```python
from build123d import *

# Parameters (mm, degrees)
SKETCH1_W           = 14.829713536
SKETCH1_H           = 33
SKETCH1_R           = 2
BOSS_EXTRUDE1_DEPTH = 4
BOSS_EXTRUDE2_DEPTH = 24


with BuildPart() as part:
    # Sketch1 → Boss-Extrude1 (new body)
    # profile 1 of 3: a face of its own
    with BuildSketch(Plane.XY):
        with Locations((7.414856768, 16.5)):
            Rectangle(SKETCH1_W, SKETCH1_H)
        with Locations((3, 2.5)):
            Circle(SKETCH1_R, mode=Mode.SUBTRACT)
        with Locations((3, 30.5)):
            Circle(SKETCH1_R, mode=Mode.SUBTRACT)
    # profile 2 of 3: a face of its own
    with BuildSketch(Plane.XY):
        Polygon((14.829713536, 33), (14.829713536, 0), (35.322939572, 0), (35.322939572, 22.058501613), (44.771529769, 22.058501613), (44.771529769, 33), align=None)
    # profile 3 of 3: a face of its own
    with BuildSketch(Plane.XY):
        Polygon((35.322939572, 22.058501613), (35.322939572, 0), (50, 0), (50, 33), (44.771529769, 33), (44.771529769, 22.058501613), align=None)
        with Locations((47, 2.5)):
            Circle(SKETCH1_R, mode=Mode.SUBTRACT)
        with Locations((47, 30.5)):
            Circle(SKETCH1_R, mode=Mode.SUBTRACT)
    extrude(amount=BOSS_EXTRUDE1_DEPTH)

    # Sketch1_3 → Boss-Extrude2 (add)
    with BuildSketch(Plane.XY):
        Polygon((14.829713536, 33), (14.829713536, 0), (35.322939572, 0), (35.322939572, 22.058501613), (44.771529769, 22.058501613), (44.771529769, 33), align=None)
    extrude(amount=BOSS_EXTRUDE2_DEPTH)


solid = part.part
```
Could you check a few things on this model? Use its own coordinates, in mm. A direction names the side the tool comes from. Round coordinates to 2 decimals unless told otherwise and drop trailing zeros. Loops run counter-clockwise (first coordinate to the right, second up) from the corner with the lowest first, then second, coordinate; pieces in that order, holes last. Notation, with made-up numbers: (34, -23) - (68, -23) arc R7 cw to (68, -10) - close; hole circle Ø2 at (66.5, 9.5). An arc over 180 degrees is marked (long way). Answer in a Markdown table with one row per item. Add a question column.
(1) If we section it at D-D (z = 5.5): Please give me the cut outline in (x, y).
(2) If we section it at A-A (y = 30.5): Please give me the cut outline in (x, z).
(3) I need wall thicknesses on line 1 along Y through (x, z) = (47, 0.9); line 2 along Z through (x, y) = (37, 18); line 3 along Y through (x, z) = (38.5, 21). Which ranges of each line are inside material? Lowest first, please.
(4) If we section it at B-B (x = 3): Please give me the cut outline in (y, z).
(5) I'm going to push flat-ended pins straight in: pin 1 (5 mm diameter, centred on x = 47, y = 2.5, fed in from +Z); pin 2 (4 mm diameter, centred on y = 28, z = 18, fed in from +X); pin 3 (3 mm diameter, centred on x = 40.5, z = 12.5, fed in from -Y). Where does each tip first touch, or does it pass through?
(6) If we mould it in two halves opening along Y, with no side actions, what happens to faces 1 (the face through (46.566, 28.548, 1.972)), 2 (the face through (40, 22.059, 14)), 3 (the face through (26, 17, 24))? For each: pulls with the +Y half, pulls with the -Y half, needs draft (parallel to the pull), parting line crosses it, or undercut.
(7) For faces 4 (the face through (35.323, 11, 14)), 5 (the face through (44.772, 27, 14)), 6 (the face through (31, 33, 9)), 7 (the face through (7, 17, 4)), 8 (the face through (0, 16, 2)), which set-ups out of +Z, -Z, +X, -X, +Y, -Y let a thin tool reach every point of the face, with its end or its side?
(8) If we section it at C-C (y = 25): Please give me the cut outline in (x, z), plus the area to 3 significant figures.
Model answer:
| question | item | result |
|---|---|---|
| 1 | outline | (14.83, 0) - (35.32, 0) - (35.32, 22.06) - (44.77, 22.06) - (44.77, 33) - (14.83, 33) - close |
| 2 | outline | (0, 0) - (1, 0) - (1, 4) - (0, 4) - close; (5, 0) - (45, 0) - (45, 4) - (44.77, 4) - (44.77, 24) - (14.83, 24) - (14.83, 4) - (5, 4) - close; (49, 0) - (50, 0) - (50, 4) - (49, 4) - close |
| 3 | line 1 | y = 0 to 0.5, 4.5 to 28.5, 32.5 to 33 |
| 3 | line 2 | z = 0 to 4 |
| 3 | line 3 | y = 22.06 to 33 |
| 4 | outline | (0, 0) - (0.5, 0) - (0.5, 4) - (0, 4) - close; (4.5, 0) - (28.5, 0) - (28.5, 4) - (4.5, 4) - close; (32.5, 0) - (33, 0) - (33, 4) - (32.5, 4) - close |
| 5 | pin 1 | stops at z = 4 |
| 5 | pin 2 | stops at x = 44.77 |
| 5 | pin 3 | stops at y = 22.06 |
| 6 | face 1 | undercut |
| 6 | face 2 | pulls with the -Y half |
| 6 | face 3 | needs draft |
| 7 | face 4 | +Z, +X, -Y |
| 7 | face 5 | +Z, +X, +Y, -Y |
| 7 | face 6 | +Z, -Z, +X, -X, +Y |
| 7 | face 7 | +Z, -X, +Y, -Y |
| 7 | face 8 | +Z, -Z, -X, +Y, -Y |
| 8 | outline | (0, 0) - (50, 0) - (50, 4) - (44.77, 4) - (44.77, 24) - (14.83, 24) - (14.83, 4) - (0, 4) - close |
| 8 | area | 799 mm² |
